For this review, take the finished solid that the model builds, in its own axes (mm). A direction names the side the tool comes from. Round coordinates to 2 decimals unless told otherwise and drop trailing zeros. Write item = value, one per line. Start each with the question number.
```python
from build123d import *

# Parameters (mm, degrees)
SKETCH_2_R               = 7.5
CUT_EXTRUDE_1_DEPTH      = 134.542128184
CUT_EXTRUDE_2_DEPTH      = 134.542128184
PATTERN_CIRCULAR_1_COUNT = 6
FILLET_1_R               = 2.5


with BuildPart() as part:
    # 草图1 → 旋转1 (revolve)
    with BuildSketch(Plane(origin=(0, 0, 0), x_dir=(0, 0, -1), z_dir=(1, 0, 0)), mode=Mode.PRIVATE) as revolve_1_sk:
        Polygon((-91.5, 33), (-91.5, 0), (-65, 0), (-65, 3), (-69, 3), (-69, 33), align=None)
    revolve(revolve_1_sk.sketch.rotate(Axis((0, 0, 0), (0, 1, 0)), 180), axis=Axis((0, 0, 0), (0, 1, 0)))

    # 草图2 → 切除-拉伸1 (cut, through all)
    with BuildSketch(Plane(origin=(0, 33, 0), x_dir=(1, 0, 0), z_dir=(0, 1, 0))):
        with Locations(Location((0, 80, 0), (0, 0, 270))):
            Circle(SKETCH_2_R)
    cut_extrude_1 = extrude(amount=-CUT_EXTRUDE_1_DEPTH, mode=Mode.SUBTRACT)

    # 草图3 → 切除-拉伸2 (cut, through all)
    with BuildSketch(Plane(origin=(0, 33, 0), x_dir=(1, 0, 0), z_dir=(0, 1, 0))):
        with BuildLine():
            Line((-72.788277417, 26.492766383), (-78.429157814, 28.545878943))
            ThreePointArc((-78.429157814, 28.545878943), (-80.374557913, 28.44634458), (-81.65798686, 26.980978151))
            ThreePointArc((-81.65798686, 26.980978151), (-86, 0), (-81.65798686, -26.980978151))
            ThreePointArc((-81.65798686, -26.980978151), (-80.374557913, -28.44634458), (-78.429157814, -28.545878943))
            Line((-78.429157814, -28.545878943), (-72.788277417, -26.492766383))
            ThreePointArc((-72.788277417, -26.492766383), (-71.394896395, -25.236492438), (-71.267736557, -23.364711127))
            ThreePointArc((-71.267736557, -23.364711127), (-75, 0), (-71.267736557, 23.364711127))
            ThreePointArc((-71.267736557, 23.364711127), (-71.394896395, 25.236492438), (-72.788277417, 26.492766383))
        make_face()
    cut_extrude_2 = extrude(amount=-CUT_EXTRUDE_2_DEPTH, mode=Mode.SUBTRACT)

    # 阵列(圆周)1: 切除-拉伸1, 切除-拉伸2 ×6 about axis
    pattern_circular_1_axis = Axis((0, 0, 0), (0, 1, 0))
    add([cut_extrude_1.rotate(pattern_circular_1_axis, i * 360 / PATTERN_CIRCULAR_1_COUNT) for i in range(1, PATTERN_CIRCULAR_1_COUNT)], mode=Mode.SUBTRACT)
    add([cut_extrude_2.rotate(pattern_circular_1_axis, i * 360 / PATTERN_CIRCULAR_1_COUNT) for i in range(1, PATTERN_CIRCULAR_1_COUNT)], mode=Mode.SUBTRACT)

    # 圆角1
    fillet_1_edges = [part.edges().sort_by_distance(p)[0] for p in [
        (0, 0, 65),
        (0, 0, 91.5),
    ]]
    fillet(fillet_1_edges, radius=FILLET_1_R)


solid = part.part
```
(1) Add section A-A on x = 36. Count the separate pieces of the cut face and the enclosed holes in it, and give its area (3 significant figures).
(2) For pin 1 Ø6 at (x, z) = (73, -7) entering from -Y; pin 2 Ø12 at (y, z) = (8, 66) entering from +X; pin 3 Ø12 at (x, z) = (-69.28, 40) entering from +Y; pin 4 Ø6 at (x, y) = (-67.5, 24.5) entering from -Z, all flat-tipped, find the tip position at first contact; note any pin that passes through.
(3) Wall thickness on L1, parallel to Z at x = -16, y = 16; L2, parallel to X at y = 20.5, z = -40; L3, parallel to Z at x = -22.5, y = 2.5: over which ranges is each line inside the solid? List them lowest first.
(4) Tool access review of faces 1 (the flat face through (41, 3, 51)), 2 (the flat face through (-61.6, 16.73, 51.69)): name each direction out of +Z, -Z, +X, -X, +Y, -Y from which nothing blocks a thin tool from reaching the whole face with its end or side.
Answer sheet:
q1.separate_pieces = 4
q1.enclosed_holes = 0
q1.area = 877 mm²
q2.pin_1 = 0
q2.pin_2 = 69.08
q2.pin_3 = through
q2.pin_4 = -64.9
q3.L1 = -90.09 to -84.07, -73.27 to -67.12, 67.12 to 73.27, 84.07 to 90.09
q3.L2 = -82.29 to -76.78, -61.78 to -56.22, 56.22 to 61.78, 76.78 to 82.29
q3.L3 = -88.69 to -83, -71.55 to -60.98, 60.98 to 71.55, 83 to 88.69
q4.face_1 = +Y
q4.face_2 = +Y, -Y
